The model under review builds one solid part; all positions refer to its coordinate system, in mm. A direction names the side the tool comes from. Coordinates: 2 decimals unless noted, no trailing zeros. Write each loop counter-clockwise with the first axis right and the second up, starting at its lowest first coordinate (ties: lowest second). Pieces come first, ordered by that corner, then holes. Notation, with made-up numbers: (72, 52) - (120, 52) arc R26 ccw to (120, 72) - close; hole circle Ø1 at (-12.5, 35). An arc over 180 degrees is marked (long way). Put each result on its own line as item: value. Start each with the question number.
Item 1: To check wall thickness, follow L1, parallel to X at y = -139.5, z = 95; L2, parallel to X at y = -42, z = 111.5; L3, parallel to X at y = 2.5, z = 136.5. State the ranges of each line that lie inside material, in increasing order. Write a range as [from, to].
Item 2: For pin 1 (3 mm diameter, centred on y = 198, z = 56, fed in from +X); pin 2 (1.5 mm diameter, centred on x = 30, z = 124.5, fed in from -Y); pin 3 (24 mm diameter, centred on y = -99, z = 65.5, fed in from -X); pin 4 (8 mm diameter, centred on x = -11, y = 183.5, fed in from -Z), all flat-tipped, find the tip position at first contact; note any pin that passes through.
Item 3: Consider section A-A on x = 0. Give the boundary of the cut face in (y, z).
Item 4: Machinability: for faces 1 (the face through (63.38, 19.96, 146.89)), 2 (the face through (-106.68, 20.14, 72.96)), which of the approach directions +Z, -Z, +X, -X, +Y, -Y give a long, thin tool a straight path to every point of the face, cutting with its end or side? Answer none if there is none.
Item 5: Consider section B-B on z = 48. State how many separate pieces and enclosed holes the cut face has, then the cut area to 3 significant figures.
Item 6: Mouldability with a two-part tool opening along Y and no side actions: class faces 3 (the face through (128.74, 4.57, 72.96)), 4 (the face through (-34.316, 64.829, 144.886)) as pulls with the +Y half, pulls with the -Y half, needs draft (parallel to the pull), parting line crosses it, or undercut.
```python
from build123d import *

# Parameters (mm, degrees)
SKETCH2_R           = 247.55
BOSS_EXTRUDE1_DEPTH = 138.9
FILLET1_R           = 10
FILLET2_R           = 10
SKETCH3_R           = 174.35
BOSS_EXTRUDE2_DEPTH = 5
CUT_EXTRUDE1_DEPTH  = 178
SKETCH9_R           = 73.351235991
BOSS_EXTRUDE3_DEPTH = 2
SKETCH10_R          = 66.449367693
BOSS_EXTRUDE4_DEPTH = 2


with BuildPart() as part:
    # Sketch2 → Boss-Extrude1 (new body)
    with BuildSketch(Plane.XY):
        Circle(SKETCH2_R)
    extrude(amount=BOSS_EXTRUDE1_DEPTH)

    # Fillet1
    fillet1_edges = [part.edges().sort_by_distance(p)[0] for p in [
        (-247.55, 0, 138.9),
    ]]
    fillet(fillet1_edges, radius=FILLET1_R)

    # Fillet2
    fillet2_edges = [part.edges().sort_by_distance(p)[0] for p in [
        (-247.55, 0, 0),
    ]]
    fillet(fillet2_edges, radius=FILLET2_R)

    # Sketch3 → Boss-Extrude2 (add)
    with BuildSketch(Plane.XY.offset(138.9)):
        Circle(SKETCH3_R)
    extrude(amount=BOSS_EXTRUDE2_DEPTH)

    # Sketch5 → Cut-Extrude1 (cut)
    with BuildSketch(Plane.XY.offset(143.9)):
        with BuildLine():
            Line((105.003706731, 43.369407929), (131.633696581, 54.021395774))
            Line((131.633696581, 54.021395774), (150.665269372, 43.031925067))
            Line((150.665269372, 43.031925067), (150.344554361, -0.360940867))
            Line((150.344554361, -0.360940867), (150.02910614, -43.041207894))
            Line((150.02910614, -43.041207894), (131.640430833, -53.657914533))
            Line((131.640430833, -53.657914533), (95.29019948, -31.084252667))
            ThreePointArc((95.29019948, -31.084252667), (106.873400183, -20.029907867), (122.363240346, -15.976029572))
            Line((122.363240346, -15.976029572), (135.299603851, 25.697677813))
            Line((135.299603851, 25.697677813), (112.925565246, 22.34468352))
            Line((112.925565246, 22.34468352), (81.592210025, -23.310129617))
            Line((81.592210025, -23.310129617), (40.25767623, 0.148769441))
            Line((40.25767623, 0.148769441), (75.177682959, 0.55093352))
            Line((75.177682959, 0.55093352), (105.003706731, 43.369407929))
        make_face()
        with BuildLine():
            Line((90.060862379, -69.251173556), (112.600749379, -86.987427346))
            Line((112.600749379, -86.987427346), (112.599374968, -108.963988211))
            Line((112.599374968, -108.963988211), (74.859693221, -130.38267383))
            Line((74.859693221, -130.38267383), (37.739773625, -151.449621172))
            Line((37.739773625, -151.449621172), (19.351098317, -140.832914533))
            Line((19.351098317, -140.832914533), (20.725347273, -98.065859815))
            ThreePointArc((20.725347273, -98.065859815), (36.090291044, -102.570033481), (47.345972712, -113.957689415))
            Line((47.345972712, -113.957689415), (89.90464373, -104.32405515))
            Line((89.90464373, -104.32405515), (75.813846191, -86.62406648))
            Line((75.813846191, -86.62406648), (20.608940598, -82.315991441))
            Line((20.608940598, -82.315991441), (20.25767623, -34.789785592))
            Line((20.25767623, -34.789785592), (38.065963903, -64.83031648))
            Line((38.065963903, -64.83031648), (90.060862379, -69.251173556))
        make_face()
        with BuildLine():
            Line((19.032947202, 141.008823121), (38.065894405, 151.995913278))
            Line((38.065894405, 151.995913278), (75.48486114, 130.021732964))
            Line((75.48486114, 130.021732964), (112.289332516, 108.408413278))
            Line((112.289332516, 108.408413278), (112.289332516, 87.175))
            Line((112.289332516, 87.175), (74.564852207, 66.981607148))
            ThreePointArc((74.564852207, 66.981607148), (70.78310914, 82.540125614), (75.017267633, 97.981659843))
            Line((75.017267633, 97.981659843), (45.394960121, 130.021732964))
            Line((45.394960121, 130.021732964), (37.111719056, 108.96875))
            Line((37.111719056, 108.96875), (60.983269426, 59.005861824))
            Line((60.983269426, 59.005861824), (20, 34.938555033))
            Line((20, 34.938555033), (37.111719056, 65.38125))
            Line((37.111719056, 65.38125), (14.942844352, 112.620581485))
            Line((14.942844352, 112.620581485), (19.032947202, 141.008823121))
        make_face()
        with BuildLine():
            Line((-14.942844352, -112.620581485), (-19.032947202, -141.008823121))
            Line((-19.032947202, -141.008823121), (-38.065894405, -151.995913278))
            Line((-38.065894405, -151.995913278), (-75.48486114, -130.021732964))
            Line((-75.48486114, -130.021732964), (-112.289332516, -108.408413278))
            Line((-112.289332516, -108.408413278), (-112.289332516, -87.175))
            Line((-112.289332516, -87.175), (-74.564852207, -66.981607148))
            ThreePointArc((-74.564852207, -66.981607148), (-70.78310914, -82.540125614), (-75.017267633, -97.981659843))
            Line((-75.017267633, -97.981659843), (-45.394960121, -130.021732964))
            Line((-45.394960121, -130.021732964), (-37.111719056, -108.96875))
            Line((-37.111719056, -108.96875), (-60.983269426, -59.005861824))
            Line((-60.983269426, -59.005861824), (-20, -34.938555033))
            Line((-20, -34.938555033), (-37.111719056, -65.38125))
            Line((-37.111719056, -65.38125), (-14.942844352, -112.620581485))
        make_face()
        with BuildLine():
            Line((-105.003706731, -43.369407929), (-131.633696581, -54.021395774))
            Line((-131.633696581, -54.021395774), (-150.665269372, -43.031925067))
            Line((-150.665269372, -43.031925067), (-150.344554361, 0.360940867))
            Line((-150.344554361, 0.360940867), (-150.02910614, 43.041207894))
            Line((-150.02910614, 43.041207894), (-131.640430833, 53.657914533))
            Line((-131.640430833, 53.657914533), (-95.29019948, 31.084252667))
            ThreePointArc((-95.29019948, 31.084252667), (-106.873400183, 20.029907867), (-122.363240346, 15.976029572))
            Line((-122.363240346, 15.976029572), (-135.299603851, -25.697677813))
            Line((-135.299603851, -25.697677813), (-112.925565246, -22.34468352))
            Line((-112.925565246, -22.34468352), (-81.592210025, 23.310129617))
            Line((-81.592210025, 23.310129617), (-40.25767623, -0.148769441))
            Line((-40.25767623, -0.148769441), (-75.177682959, -0.55093352))
            Line((-75.177682959, -0.55093352), (-105.003706731, -43.369407929))
        make_face()
        with BuildLine():
            Line((-90.060862379, 69.251173556), (-112.600749379, 86.987427346))
            Line((-112.600749379, 86.987427346), (-112.599374968, 108.963988211))
            Line((-112.599374968, 108.963988211), (-74.859693221, 130.38267383))
            Line((-74.859693221, 130.38267383), (-37.739773625, 151.449621172))
            Line((-37.739773625, 151.449621172), (-19.351098317, 140.832914533))
            Line((-19.351098317, 140.832914533), (-20.725347273, 98.065859815))
            ThreePointArc((-20.725347273, 98.065859815), (-36.090291044, 102.570033481), (-47.345972712, 113.957689415))
            Line((-47.345972712, 113.957689415), (-89.90464373, 104.32405515))
            Line((-89.90464373, 104.32405515), (-75.813846191, 86.62406648))
            Line((-75.813846191, 86.62406648), (-20.608940598, 82.315991441))
            Line((-20.608940598, 82.315991441), (-20.25767623, 34.789785592))
            Line((-20.25767623, 34.789785592), (-38.065963903, 64.83031648))
            Line((-38.065963903, 64.83031648), (-90.060862379, 69.251173556))
        make_face()
    extrude(amount=-CUT_EXTRUDE1_DEPTH, mode=Mode.SUBTRACT)

    # Sketch9 → Boss-Extrude3 (add)
    with BuildSketch(Plane.XY.offset(143.9)):
        with Locations(Location((0, 0, 0), (0, 0, 180.413898519))):
            Circle(SKETCH9_R)
    extrude(amount=BOSS_EXTRUDE3_DEPTH)

    # Sketch10 → Boss-Extrude4 (add)
    with BuildSketch(Plane.XY.offset(145.9)):
        Circle(SKETCH10_R)
    extrude(amount=BOSS_EXTRUDE4_DEPTH)


solid = part.part
```
Report:
1. L1: [-204.5, -59.34], [-18.82, 19.39], [58.79, 204.5]
1. L2: [-243.96, -150.66], [-104.05, -32.02], [-23.97, 20.31], [24.53, 112.87], [150.04, 243.96]
1. L3: [-244.04, -150.33], [-126.55, -95.87], [-44.92, 76.54], [99.31, 128.1], [150.37, 244.04]
2. pin 1: x = 150.56
2. pin 2: y = -245.82
2. pin 3: x = -231.76
2. pin 4: z = 0
3. outline: (-247.55, 10) arc R10 ccw to (-237.55, 0) - (237.55, 0) arc R10 ccw to (247.55, 10) - (247.55, 128.9) arc R10 ccw to (237.55, 138.9) - (174.35, 138.9) - (174.35, 143.9) - (73.35, 143.9) - (73.35, 145.9) - (66.45, 145.9) - (66.45, 147.9) - (-66.45, 147.9) - (-66.45, 145.9) - (-73.35, 145.9) - (-73.35, 143.9) - (-174.35, 143.9) - (-174.35, 138.9) - (-237.55, 138.9) arc R10 ccw to (-247.55, 128.9) - close
4. face 1: +Z
4. face 2: +Z, -Z
5. separate pieces: 1
5. enclosed holes: 6
5. area: 164,000 mm²
6. face 3: undercut
6. face 4: parting line crosses it
